Could you check a few things on this drawing? It's one solid part, dimensions in mm from its lowest x, y, z. Give positions to 0.01 mm unless a question says otherwise; leave off trailing zeros. Order: outer loops, then holes, each group sorted by start corner. A loop starts at its lowest first (then second) coordinate and runs counter-clockwise, first axis right, second up. Notation, with made-up numbers: (76, 15) - (101, 15) arc R11 ccw to (101, 26) - close; hole circle Ø1 at (35, -14). An arc over 180 degrees is marked (long way). One line per question, with ' | ' between items. Start each with the question number.
1. I need wall thicknesses on probe 1 along Z at (x, y) = (86, 3.5); probe 2 along X at (y, z) = (5, 36); probe 3 along Z at (x, y) = (74, 1). Which ranges of each line are inside material? Lowest first, please. Write a range as from..to.
2. Imagine slicing it at B-B (x = 73). Please give me the cut outline in (y, z).
3. Imagine slicing it at A-A (z = 25). Please give me the cut outline in (x, y), and give its area (3 significant figures).
4. If we mould it in two halves opening along X, with no side actions, what happens to the marked faces 1, 2 and 3? For each: released by +X, released by -X, zero draft, split by the parting line, or undercut.
5. For P1, Ø4, axis at y = 8.5, z = 50, coming from the -X side, with a flat end and sliding along its axis, tell me the tip position at first contact or that it passes through.
6. Imagine slicing it at C-C (z = 45). Please give me the cut outline in (x, y).
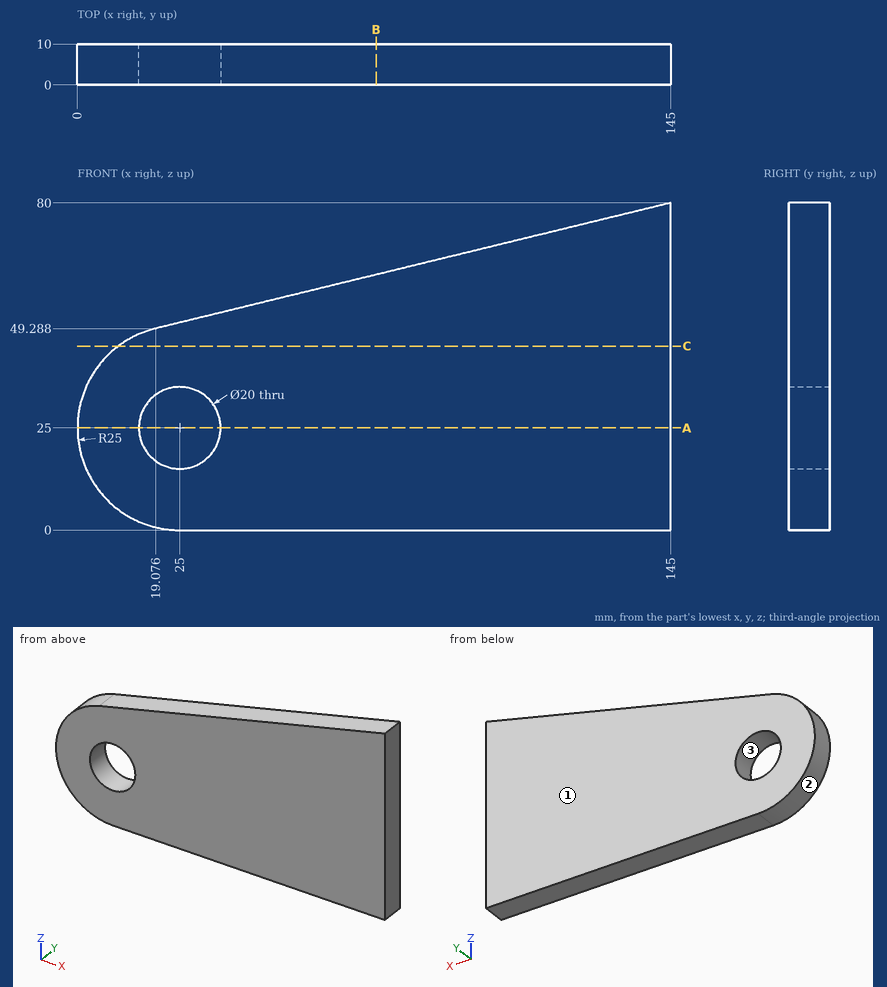
Results found:
1) probe 1: z = 0..65.61 | probe 2: x = 2.55..145 | probe 3: z = 0..62.68
2) outline: (0, 0) - (10, 0) - (10, 62.44) - (0, 62.44) - close
3) outline: (0, 0) - (15, 0) - (15, 10) - (0, 10) - close; (35, 0) - (145, 0) - (145, 10) - (35, 10) - close | area: 1,250 mm2
4) face 1: zero draft | face 2: released by -X | face 3: undercut
5) P1: stops at x = 15.2
6) outline: (10, 0) - (145, 0) - (145, 10) - (10, 10) - close
